from build123d import *

# Parameters (mm, degrees)
EXTRUDE_1_DEPTH      = 18.35
FILLET_1_R           = 0.7
SHELL_START          = -28.75
SHELL_1_OUTLINE_W    = 32.7
SHELL_1_OUTLINE_H    = 34.5
SHELL_1_DEPTH        = 57.5
SHELL_START_2        = -42
SHELL_1_2_OUTLINE_W  = 32.7
SHELL_1_2_OUTLINE_H  = 15.5
SHELL_1_2_DEPTH      = 84
SHELL_START_3        = -21.75
SHELL_1_3_OUTLINE_W  = 32.7
SHELL_1_3_OUTLINE_H  = 8.5
SHELL_1_3_DEPTH      = 43.5
SKETCH_2_W           = 32
SKETCH_2_H           = 43
CUT_EXTRUDE_1_DEPTH  = 1.5
SKETCH_7_W           = 25.5
SKETCH_7_H           = 2
SKETCH_7_W_2         = 26
CUT_EXTRUDE_5_DEPTH  = 11
SKETCH_8_W           = 2.7
SKETCH_8_H           = 7
CUT_EXTRUDE_6_DEPTH  = 36
SKETCH_9_W           = 26
SKETCH_9_H           = 5
CUT_EXTRUDE_7_DEPTH  = 0.5
SKETCH_10_W          = 34.7
SKETCH_10_H          = 86
SKETCH_10_W_2        = 32.7
SKETCH_10_H_2        = 84
CUT_EXTRUDE_8_DEPTH  = 1.5
SKETCH_11_W          = 2.5
SKETCH_11_H          = 11
CUT_EXTRUDE_9_DEPTH  = 2
SKETCH_12_R          = 1.6
SKETCH_12_R_2        = 3.1
CUT_EXTRUDE_10_DEPTH = 2
EXTRUDE_2_REACH      = 72.956


# Read off the part's stored shape, not the designer's step: Оболочка1
with BuildPart() as part:
    # Эскиз1 → Вытянуть1 (new, symmetric)
    with BuildSketch(Plane(origin=(0, 0, 0), x_dir=(0, 0, -1), z_dir=(1, 0, 0))):
        Polygon((-17.5, -30.75), (-17.5, -44), (0, -44), (0, 44), (-17.5, 44), (-17.5, 30.75), (-36.5, 30.75), (-36.5, 23.75), (-46, 23.75), (-46, -23.75), (-36.5, -23.75), (-36.5, -30.75), align=None)
    extrude(amount=EXTRUDE_1_DEPTH, both=True)

    # Скругление1
    fillet_1_edges = [part.edges().sort_by_distance(p)[0] for p in [
        (18.35, 37.375, 17.5),
        (-18.35, -37.375, 17.5),
        (-18.35, -30.75, 27),
        (-18.35, -27.25, 36.5),
        (-18.35, -23.75, 41.25),
        (-18.35, 0, 46),
        (-18.35, 23.75, 41.25),
        (-18.35, 27.25, 36.5),
        (-18.35, 30.75, 27),
        (18.35, 30.75, 27),
        (-18.35, 37.375, 17.5),
        (-18.35, 44, 8.75),
        (18.35, 27.25, 36.5),
        (0, -44, 17.5),
        (0, -30.75, 36.5),
        (0, -23.75, 46),
        (0, 23.75, 46),
        (18.35, 23.75, 41.25),
        (0, 30.75, 36.5),
        (0, 44, 17.5),
        (18.35, 0, 46),
        (18.35, -23.75, 41.25),
        (18.35, -27.25, 36.5),
        (18.35, -30.75, 27),
        (18.35, -37.375, 17.5),
        (18.35, -44, 8.75),
        (18.35, 44, 8.75),
        (-18.35, -44, 8.75),
    ]]
    fillet(fillet_1_edges, radius=FILLET_1_R)

    # Оболочка1 outline → Оболочка1 (cut)
    with BuildSketch(Plane(origin=(0, 0, 0), x_dir=(1, 0, 0), z_dir=(0, 1, 0)).offset(SHELL_START)):
        with Locations((0, -17.25)):
            Rectangle(SHELL_1_OUTLINE_W, SHELL_1_OUTLINE_H)
    extrude(amount=SHELL_1_DEPTH, mode=Mode.SUBTRACT)

    # Shell 1 2 outline → Shell 1 2 (cut)
    with BuildSketch(Plane(origin=(0, 0, 0), x_dir=(1, 0, 0), z_dir=(0, 1, 0)).offset(SHELL_START_2)):
        with Locations((0, -7.75)):
            Rectangle(SHELL_1_2_OUTLINE_W, SHELL_1_2_OUTLINE_H)
    extrude(amount=SHELL_1_2_DEPTH, mode=Mode.SUBTRACT)

    # Shell 1 3 outline → Shell 1 3 (cut)
    with BuildSketch(Plane(origin=(0, 0, 0), x_dir=(1, 0, 0), z_dir=(0, 1, 0)).offset(SHELL_START_3)):
        with Locations((0, -38.75)):
            Rectangle(SHELL_1_3_OUTLINE_W, SHELL_1_3_OUTLINE_H)
    extrude(amount=SHELL_1_3_DEPTH, mode=Mode.SUBTRACT)

    # Эскиз2 → Вырез-Вытянуть1 (cut)
    with BuildSketch(Plane.XY.offset(46)):
        Rectangle(SKETCH_2_W, SKETCH_2_H)
    extrude(amount=-CUT_EXTRUDE_1_DEPTH, mode=Mode.SUBTRACT)

    # Эскиз7 → Вырез-Вытянуть5 (cut)
    with BuildSketch(Plane(origin=(0, 0, 0), x_dir=(-1, 0, 0), z_dir=(0, 0, -1))):
        with Locations((0, -43)):
            Rectangle(SKETCH_7_W, SKETCH_7_H)
        with Locations((0, 43)):
            Rectangle(SKETCH_7_W_2, SKETCH_7_H)
    extrude(amount=-CUT_EXTRUDE_5_DEPTH, mode=Mode.SUBTRACT)

    # Эскиз8 → Вырез-Вытянуть6 (cut, symmetric)
    with BuildSketch(Plane(origin=(0, 0, 0), x_dir=(0, 0, -1), z_dir=(1, 0, 0))):
        with Locations((-5.35, 0)):
            Rectangle(SKETCH_8_W, SKETCH_8_H)
    extrude(amount=CUT_EXTRUDE_6_DEPTH, both=True, mode=Mode.SUBTRACT)

    # Эскиз9 → Вырез-Вытянуть7 (cut)
    with BuildSketch(Plane.XY.offset(17.5)):
        with Locations((0, 38.5)):
            Rectangle(SKETCH_9_W, SKETCH_9_H)
    cut_extrude_7 = extrude(amount=-CUT_EXTRUDE_7_DEPTH, mode=Mode.SUBTRACT)

    # Зеркальное отражение1: Вырез-Вытянуть7 across plane
    add(cut_extrude_7.mirror(Plane.ZX), mode=Mode.SUBTRACT)

    # Эскиз10 → Вырез-Вытянуть8 (cut)
    with BuildSketch(Plane(origin=(0, 0, 0), x_dir=(-1, 0, 0), z_dir=(0, 0, -1))):
        Rectangle(SKETCH_10_W, SKETCH_10_H)
        Rectangle(SKETCH_10_W_2, SKETCH_10_H_2, mode=Mode.SUBTRACT)
    extrude(amount=-CUT_EXTRUDE_8_DEPTH, mode=Mode.SUBTRACT)

    # Эскиз11 → Вырез-Вытянуть9 (cut)
    with BuildSketch(Plane.XZ.offset(44)):
        with Locations((-14, 5.5)):
            Rectangle(SKETCH_11_W, SKETCH_11_H)
    extrude(amount=-CUT_EXTRUDE_9_DEPTH, mode=Mode.SUBTRACT)

    # Эскиз12 → Вырез-Вытянуть10 (cut)
    with BuildSketch(Plane.XY.offset(44.5)):
        with Locations((-8.5, 17.790145453)):
            Circle(SKETCH_12_R)
        with Locations((-8.5, 12.29)):
            Circle(SKETCH_12_R)
        with Locations((8.5, 12.29)):
            Circle(SKETCH_12_R)
        with Locations((9, -14.5)):
            Circle(SKETCH_12_R_2)
    extrude(amount=-CUT_EXTRUDE_10_DEPTH, mode=Mode.SUBTRACT)

    # Эскиз13 → Вытянуть2 (add, up to next)
    with BuildSketch(Plane(origin=(-13, 0, 0), x_dir=(0, 0, -1), z_dir=(1, 0, 0)), mode=Mode.PRIVATE) as extrude_2_sk1:
        Polygon((-11, 44), (-11, 42), (-1.508482634, 42), (-1.5, 43), (0, 43), (0, 44), align=None)
    extrude_2_tool1 = extrude(extrude_2_sk1.sketch, amount=EXTRUDE_2_REACH, mode=Mode.PRIVATE) - part.part
    add(extrude_2_tool1.solids().sort_by_distance((-13, 43.036731, 5.84846))[0])


solid = part.part
Input: part model. Units: mm. Frame: model coordinates. A direction names the side the tool comes from. Give positions to 0.01 mm unless a question says otherwise; leave off trailing zeros. Order: outer loops, then holes, each group sorted by start corner. A loop starts at its lowest first (then second) coordinate and runs counter-clockwise, first axis right, second up. Notation, with made-up numbers: (35, 62.25) - (83, 62.25) arc R21 ccw to (83, 90.25) - close; hole circle Ø9 at (48.5, -34.5). An arc over 180 degrees is marked (long way). Answer as a JSON object with one key per item and string values. Group by question number.
Q1. Mould query, pull axis Y, two halves, no side actions, for faces 1 (the face through (0, -30.75, 27)), 2 (the face through (0, 30.75, 27)), 3 (the face through (0, -27, 36.5)), 4 (the face through (0, -35, 15.5)). Classes: pulls with the +Y half, pulls with the -Y half, needs draft (parallel to the pull), parting line crosses it, or undercut.
Q2. Set-up query: faces 5 (the face through (0, 0, 44.5)), 6 (the face through (-17, 2, 46)), 7 (the face through (-1, -43, 11)), 8 (the face through (0, 21.75, 39)), 9 (the face through (17, -3.5, 5)). Return all of +Z, -Z, +X, -X, +Y, -Y with unobstructed straight access to the full face (end or side cutting, diameter ignored); none if empty.
Q3. Cut plane C-C, the plane z = 5.5. Output: boundary loops of the cut face in (x, y), then the cut area to 3 significant figures.
Q4. Cut plane D-D, the plane z = 31. Output: boundary loops of the cut face in (x, y).
Q5. Line query: probe 1 along Y at (x, z) = (-8.5, 44); probe 2 along X at (y, z) = (-17.5, 11); probe 3 along Y at (x, z) = (9, 43.5). Output: solid intervals per line, ascending.
Q6. Cut plane A-A, the plane y = 12.29. Output: boundary loops of the cut face in (x, z).
Q7. Cut plane B-B, the plane y = -14.5. Output: boundary loops of the cut face in (x, z).
Q8. First-contact query: pin 1 Ø12 at (x, z) = (5, 34.5) entering from +Y; pin 2 Ø1.6 at (x, z) = (8, 1) entering from -Y; pin 3 Ø12 at (x, y) = (-4, 29.5) entering from -Z. Flat tips, straight axial feed; report the tip coordinate or a pass-through.
Results:
{
 "1": {"face 1": "pulls with the -Y half", "face 2": "pulls with the +Y half", "face 3": "needs draft", "face 4": "undercut"},
 "2": {"face 5": "+Z", "face 6": "+Z, +X, -X, +Y, -Y", "face 7": "-Z, -Y", "face 8": "-Z", "face 9": "+X, -X"},
 "3": {"outline": "(-18.35, -43.3) arc R0.7 ccw to (-17.65, -44) - (-15.25, -44) - (-15.25, -42) - (-16.35, -42) - (-16.35, -3.5) - (-18.35, -3.5) - close; (-18.35, 3.5) - (-16.35, 3.5) - (-16.35, 42) - (16.35, 42) - (16.35, 3.5) - (18.35, 3.5) - (18.35, 43.3) arc R0.7 ccw to (17.65, 44) - (-17.65, 44) arc R0.7 ccw to (-18.35, 43.3) - close; (12.75, -44) - (17.65, -44) arc R0.7 ccw to (18.35, -43.3) - (18.35, -3.5) - (16.35, -3.5) - (16.35, -42) - (12.75, -42) - close", "area": "398 mm^2"},
 "4": {"outline": "(-18.35, -30.05) arc R0.7 ccw to (-17.65, -30.75) - (17.65, -30.75) arc R0.7 ccw to (18.35, -30.05) - (18.35, 30.05) arc R0.7 ccw to (17.65, 30.75) - (-17.65, 30.75) arc R0.7 ccw to (-18.35, 30.05) - close; hole (-16.35, -28.75) - (16.35, -28.75) - (16.35, 28.75) - (-16.35, 28.75) - close"},
 "5": {"probe 1": "-23.75 to 10.69, 13.89 to 16.19, 19.39 to 23.75", "probe 2": "-18.35 to -16.35, 16.35 to 18.35", "probe 3": "-23.75 to -17.6, -11.4 to 10.77, 13.81 to 23.75"},
 "6": {"outline": "(-18.35, 0) - (-17.35, 0) - (-17.35, 1.5) - (-16.35, 1.5) - (-16.35, 43) - (-10.1, 43) - (-10.1, 44.5) - (-16, 44.5) - (-16, 46) - (-17.65, 46) arc R0.7 ccw to (-18.35, 45.3) - close; (-6.9, 43) - (6.9, 43) - (6.9, 44.5) - (-6.9, 44.5) - close; (10.1, 43) - (16.35, 43) - (16.35, 1.5) - (17.35, 1.5) - (17.35, 0) - (18.35, 0) - (18.35, 45.3) arc R0.7 ccw to (17.65, 46) - (16, 46) - (16, 44.5) - (10.1, 44.5) - close"},
 "7": {"outline": "(-18.35, 0) - (-17.35, 0) - (-17.35, 1.5) - (-16.35, 1.5) - (-16.35, 43) - (5.9, 43) - (5.9, 44.5) - (-16, 44.5) - (-16, 46) - (-17.65, 46) arc R0.7 ccw to (-18.35, 45.3) - close; (12.1, 43) - (16.35, 43) - (16.35, 1.5) - (17.35, 1.5) - (17.35, 0) - (18.35, 0) - (18.35, 45.3) arc R0.7 ccw to (17.65, 46) - (16, 46) - (16, 44.5) - (12.1, 44.5) - close"},
 "8": {"pin 1": "y = 30.75", "pin 2": "y = 42", "pin 3": "z = 15.5"}
}
